Verification items for this drawing (mm, ordinates from the low corner). A direction names the side the tool comes from. Give positions to 0.01 mm unless a question says otherwise; leave off trailing zeros. Order: outer loops, then holes, each group sorted by start corner. A loop starts at its lowest first (then second) coordinate and runs counter-clockwise, first axis right, second up. Notation, with made-up numbers: (-10.75, 41) -> (4.25, 41) arc R21 ccw to (4.25, 75) -> close; hole circle Ø3 at (39.25, 25.5). An arc over 180 degrees is marked (long way). One line per question, with ' | ' between items.
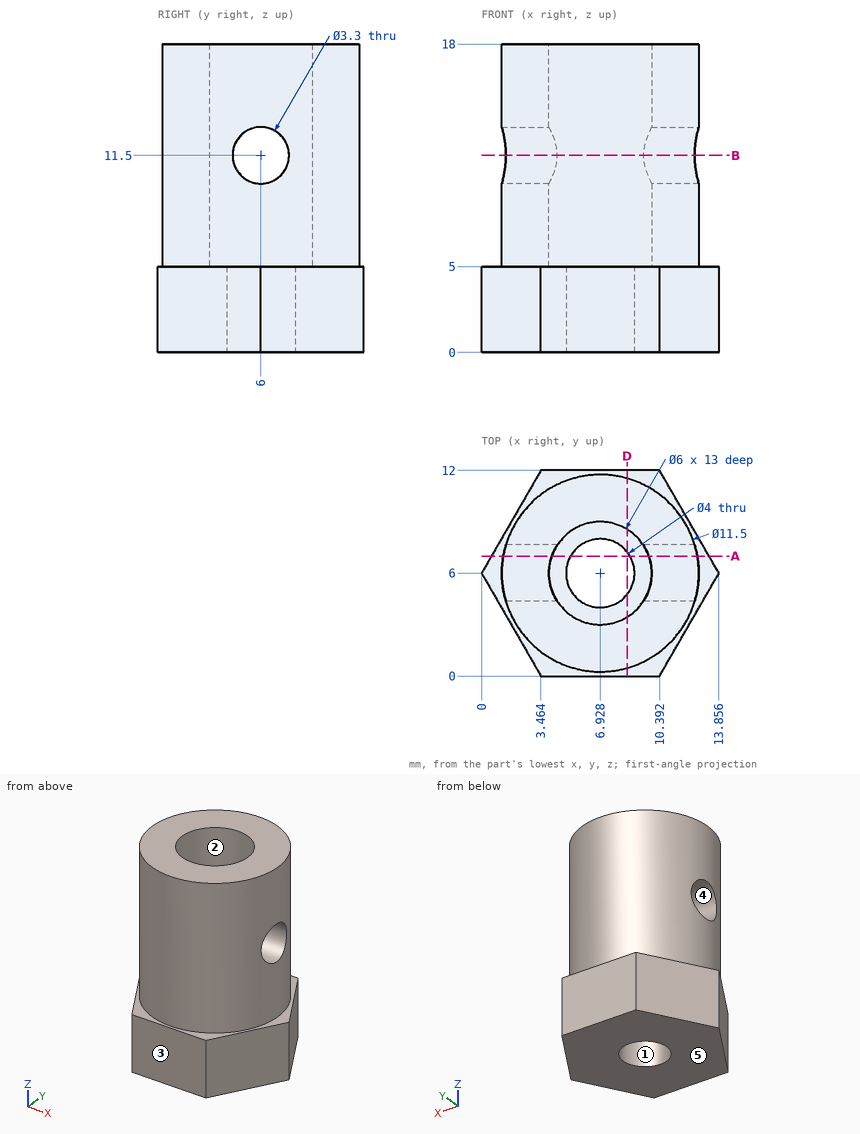
Q1. Thickness scan on line 1 (Y direction, x = 7, z = 12.25); line 2 (Z direction, x = 3.5, y = 0.5); line 3 (X direction, y = 4.25, z = 1.25) (1 decimal). Record the ranges inside material, lowest first.
Result sheet:
line 1: y = 0.25 to 3, 9 to 11.75 | line 2: z = 0 to 5 | line 3: x = 1 to 6, 7.9 to 12.8
Q2. Section check D-D (x = 8.5). Enter the section's corners in (y, z) (1 decimal).
Result sheet:
outline: (0, 0) -> (4.8, 0) -> (4.8, 5) -> (3.4, 5) -> (3.4, 18) -> (0.5, 18) -> (0.5, 5) -> (0, 5) -> close; (7.2, 0) -> (12, 0) -> (12, 5) -> (11.5, 5) -> (11.5, 18) -> (8.6, 18) -> (8.6, 5) -> (7.2, 5) -> close
Q3. Access from +Z, -Z, +X, -X, +Y, -Y to the whole of each face (thin tool, end or side, straight path). Record for the marked faces 1 and 2.
Result sheet:
face 1: +Z, -Z | face 2: +Z
Q4. Section check A-A (y = 7). Enter the section's corners in (x, z), and give its area (3 significant figures).
Result sheet:
outline: (0.58, 0) -> (5.2, 0) -> (5.2, 5) -> (4.1, 5) -> (4.1, 10.19) -> (1.27, 10.19) -> (1.27, 5) -> (0.58, 5) -> close; (1.27, 12.81) -> (4.1, 12.81) -> (4.1, 18) -> (1.27, 18) -> close; (8.66, 0) -> (13.28, 0) -> (13.28, 5) -> (12.59, 5) -> (12.59, 10.19) -> (9.76, 10.19) -> (9.76, 5) -> (8.66, 5) -> close; (9.76, 12.81) -> (12.59, 12.81) -> (12.59, 18) -> (9.76, 18) -> close | area: 105 mm2
Q5. Depth check by flat-ended pin: pin 1 Ø5.5 at (x, y) = (6.93, 6) entering from +Z; pin 2 Ø5 at (x, z) = (5, 10.5) entering from -Y; pin 3 Ø3 at (y, z) = (7, 15) entering from -X. Enter the tip coordinate at first touch or a pass-through.
Result sheet:
pin 1: stops at z = 5 | pin 2: stops at y = 0.25 | pin 3: stops at x = 1.18
Q6. Mould release check, pull along Z, two halves, no side actions. Record for the marked faces 3, 4 and 5: pulls with the +Z half, pulls with the -Z half, needs draft (parallel to the pull), parting line crosses it, or undercut.
Result sheet:
face 3: needs draft | face 4: undercut | face 5: pulls with the -Z half
Q7. Section check B-B (z = 11.5). Enter the section's corners in (x, y).
Result sheet:
outline: (1.42, 4.35) arc R5.75 ccw to (12.44, 4.35) -> (9.43, 4.35) arc R3 cw to (4.42, 4.35) -> close; (1.42, 7.65) -> (4.42, 7.65) arc R3 cw to (9.43, 7.65) -> (12.44, 7.65) arc R5.75 ccw to start
